Read the model definition and answer for the solid it produces. Units are mm, in the model's axes. A direction names the side the tool comes from. Coordinates: 2 decimals unless noted, no trailing zeros. Write each loop counter-clockwise with the first axis right and the second up, starting at its lowest first coordinate (ties: lowest second). Pieces come first, ordered by that corner, then holes.
(1) The part is cut by section D-D, the plane y = -6.5. Determine the outline of the cut face in (x, z) (3 decimals).
(2) Which of the six approach directions +Z, -Z, +X, -X, +Y, -Y give full straight-line access (tool end or side, diameter ignored) to faces 1 (the flat face through (1, -6, 0.07)), 2 (the flat face through (2.78, 0, 1)), 3 (the flat face through (2.3, 0, 1)), 4 (the flat face through (-0.24, 0, 1))?
(3) Straight lines are drawn through the part: line 1 along Y through (x, z) = (0.05, 0.75); line 2 along Y through (x, z) = (-0.1, 2.5); line 3 along Y through (x, z) = (-0.15, -1.75). For each, find the intervals that lie inside material, in ascending order.
(4) The part is cut by section B-B, the plane z = 1. Determine the outline of the cut face in (x, y).
(5) The part is cut by section A-A, the plane z = -0.25. Determine the outline of the cut face in (x, y), and give its area (3 significant figures).
(6) The part is cut by section C-C, the plane x = 2.6. Determine the outline of the cut face in (y, z), and give its area (3 significant figures).
(7) Given pin 1 (1.2 mm diameter, centred on x = 2, y = -6, fed in from -Z); pin 2 (0.5 mm diameter, centred on x = 2.5, z = -1, fed in from -Y); pin 3 (0.5 mm diameter, centred on x = 0, y = -3, fed in from +Z), each flat-ended and moving along its own axis, determine where each tip first touches the part or whether it passes through.
```python
from build123d import *

# Parameters (mm, degrees)
PAD_DEPTH    = 4.8
SKETCH002_W  = 0.48
SKETCH002_H  = 4.3
PAD002_DEPTH = 0.38
FILLET_R     = 0.35
SKETCH001_W  = 0.48
SKETCH001_H  = 0.38
PAD001_DEPTH = 4


with BuildPart() as pad:
    # Sketch → Pad (new body)
    with BuildSketch(Plane(origin=(0, -4, 1.4), x_dir=(1, 0, 0), z_dir=(0, -1, 0))):
        with BuildLine():
            Line((-0.745769, -1.33), (3.285769, -1.33))
            ThreePointArc((3.285769, -1.33), (1.27, 2.415), (-0.745769, -1.33))
        make_face()
    extrude(amount=PAD_DEPTH)


with BuildPart() as fillet_body:
    # Sketch002 → Pad002 (new body)
    with BuildSketch(Plane.XY.offset(1.4)):
        with Locations((2.54, -1.96)):
            Rectangle(SKETCH002_W, SKETCH002_H)
        with Locations((0, -1.96)):
            Rectangle(SKETCH002_W, SKETCH002_H)
    extrude(amount=PAD002_DEPTH)

    # Fillet
    fillet_edges = [fillet_body.edges().sort_by_distance(p)[0] for p in [
        (2.54, 0.19, 1.78),
        (0, 0.19, 1.78),
    ]]
    fillet(fillet_edges, radius=FILLET_R)


with BuildPart() as obj1:
    # Sketch001 → Pad001 (new body)
    with BuildSketch(Plane.XY.offset(1.4)):
        Rectangle(SKETCH001_W, SKETCH001_H)
        with Locations((2.54, 0)):
            Rectangle(SKETCH001_W, SKETCH001_H)
    extrude(amount=-PAD001_DEPTH)

    add(pad.part)
    add(fillet_body.part)


solid = obj1.part
```
Computed:
1. outline: (-0.746, 0.07) - (3.286, 0.07) arc R2.415 ccw (long way) to start
2. face 1: -Z, +X, -X, -Y
2. face 2: +Z, -Z, +X, +Y
2. face 3: +Z, -Z, +Y
2. face 4: +Z, -Z, -X, +Y
3. line 1: y = -8.8 to -4, -0.19 to 0.19
3. line 2: y = -8.8 to -4
3. line 3: y = -0.19 to 0.19
4. outline: (-1.11, -8.8) - (3.65, -8.8) - (3.65, -4) - (-1.11, -4) - close; (-0.24, -0.19) - (0.24, -0.19) - (0.24, 0.19) - (-0.24, 0.19) - close; (2.3, -0.19) - (2.78, -0.19) - (2.78, 0.19) - (2.3, 0.19) - close
5. outline: (-0.24, -0.19) - (0.24, -0.19) - (0.24, 0.19) - (-0.24, 0.19) - close; (2.3, -0.19) - (2.78, -0.19) - (2.78, 0.19) - (2.3, 0.19) - close
5. area: 0.365 mm2
6. outline: (-8.8, 0.07) - (-4, 0.07) - (-4, 1.4) - (-0.19, 1.4) - (-0.19, -2.6) - (0.19, -2.6) - (0.19, 1.43) arc R0.35 ccw to (-0.16, 1.78) - (-4, 1.78) - (-4, 3.42) - (-8.8, 3.42) - close
6. area: 19.1 mm2
7. pin 1: stops at z = 0.07
7. pin 2: stops at y = -0.19
7. pin 3: stops at z = 1.78
